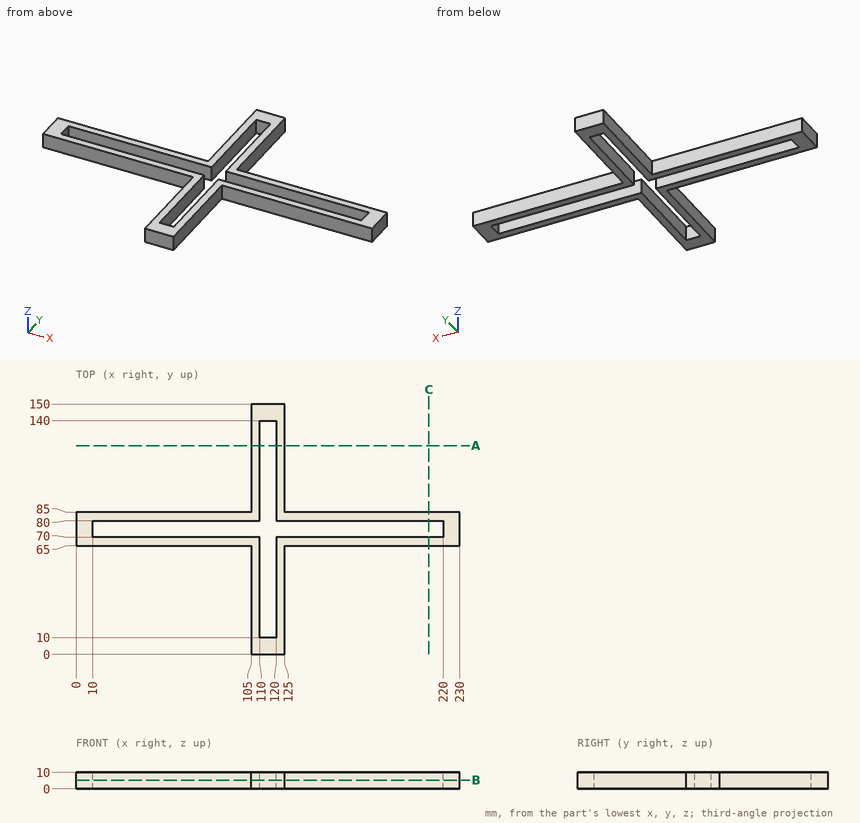
Geometry check sheet. Reference: drawing and pictorial views, mm from the part's lowest x, y, z. Round coordinates to 2 decimals unless told otherwise and drop trailing zeros. Loops run counter-clockwise (first coordinate to the right, second up) from the corner with the lowest first, then second, coordinate; pieces in that order, holes last. Notation, with made-up numbers: (59.25, 62.5) -> (107.25, 62.5) arc R19 cw to (107.25, 97.5) -> close; hole circle Ø9 at (2.25, 5.5). An arc over 180 degrees is marked (long way). Answer as a JSON object with one key per item and string values.
Q1. Scan lines: line 1 (X direction, y = 136.5, z = 6); line 2 (Y direction, x = 90, z = 2); line 3 (X direction, y = 141, z = 4.5). Record each from-to range of solid material in increasing order. Write a range as from..to.
Data:
{"line 1": "x = 105..110, 120..125", "line 2": "y = 65..70, 80..85", "line 3": "x = 105..125"}
Q2. Section check C-C (x = 211.5). Record the boundary of the cut face in (y, z).
Data:
{"outline": "(65, 0) -> (70, 0) -> (70, 10) -> (65, 10) -> close; (80, 0) -> (85, 0) -> (85, 10) -> (80, 10) -> close"}
Q3. Go/stop test with flat-tipped pins: P1, Ø1.5, axis at y = 56, z = 4.5, coming from the +X side; P2, Ø2, axis at x = 78, z = 8.5, coming from the +Y side; P3, Ø5, axis at x = 190.5, z = 6, coming from the -Y side. Record where each tip stops, or that it passes through.
Data:
{"P1": "stops at x = 125", "P2": "stops at y = 85", "P3": "stops at y = 65"}
Q4. Section check B-B (z = 5.25). Record the boundary of the cut face in (x, y).
Data:
{"outline": "(0, 65) -> (105, 65) -> (105, 0) -> (125, 0) -> (125, 65) -> (230, 65) -> (230, 85) -> (125, 85) -> (125, 150) -> (105, 150) -> (105, 85) -> (0, 85) -> close; hole (10, 70) -> (110, 70) -> (110, 10) -> (120, 10) -> (120, 70) -> (220, 70) -> (220, 80) -> (120, 80) -> (120, 140) -> (110, 140) -> (110, 80) -> (10, 80) -> close"}
Q5. Section check A-A (y = 125). Record the boundary of the cut face in (x, z), then the cut area to 3 significant figures.
Data:
{"outline": "(105, 0) -> (110, 0) -> (110, 10) -> (105, 10) -> close; (120, 0) -> (125, 0) -> (125, 10) -> (120, 10) -> close", "area": "100 mm2"}
